from build123d import *

# Parameters (mm, degrees)
CUT_EXTRUDE3_START = 21
CUT_EXTRUDE3_DEPTH = 6.2


with BuildPart() as part:
    # Sketch1 → Revolve1 (revolve)
    with BuildSketch(Plane.XY, mode=Mode.PRIVATE) as revolve1_sk:
        with BuildLine():
            Line((24.3, 17.078694854), (5.260372827, 17.078694854))
            Line((5.260372827, 17.078694854), (5.260372827, 16.028694854))
            Line((5.260372827, 16.028694854), (3.960372827, 16.028694854))
            Line((3.960372827, 16.028694854), (3.960372827, 17.078694854))
            Line((3.960372827, 17.078694854), (-0.7, 17.078694854))
            Line((-0.7, 17.078694854), (-0.7, 2.078694854))
            Line((-0.7, 2.078694854), (295.3, 2.078694854))
            Line((295.3, 2.078694854), (295.3, 17.078694854))
            Line((295.3, 17.078694854), (290.659722162, 17.078694854))
            Line((290.659722162, 17.078694854), (290.659722162, 16.028694854))
            Line((290.659722162, 16.028694854), (289.359722162, 16.028694854))
            Line((289.359722162, 16.028694854), (289.359722162, 17.078694854))
            Line((289.359722162, 17.078694854), (270.3, 17.078694854))
            Line((270.3, 17.078694854), (270.3, 19.578694854))
            Line((270.3, 19.578694854), (229.3, 19.578694854))
            Line((229.3, 19.578694854), (229.3, 18.528694854))
            Line((229.3, 18.528694854), (228, 18.528694854))
            Line((228, 18.528694854), (228, 19.578694854))
            Line((228, 19.578694854), (178, 19.578694854))
            Line((178, 19.578694854), (178, 22.078694854))
            Line((178, 22.078694854), (76.4, 22.078694854))
            Line((76.4, 22.078694854), (76.4, 19.578694854))
            Line((76.4, 19.578694854), (36.4, 19.578694854))
            Line((36.4, 19.578694854), (36.4, 18.728694854))
            ThreePointArc((36.4, 18.728694854), (36.341421356, 18.587273498), (36.2, 18.528694854))
            Line((36.2, 18.528694854), (35.2, 18.528694854))
            ThreePointArc((35.2, 18.528694854), (35.058578644, 18.587273498), (35, 18.728694854))
            Line((35, 18.728694854), (35, 19.578694854))
            Line((35, 19.578694854), (24.3, 19.578694854))
            Line((24.3, 19.578694854), (24.3, 17.078694854))
        make_face()
    revolve(revolve1_sk.sketch.rotate(Axis((-34.240282719, 2.078694854, 0), (1, 0, 0)), 180), axis=Axis((-34.240282719, 2.078694854, 0), (1, 0, 0)))

    # Sketch4 → Cut-Extrude3 (cut)
    with BuildSketch(Plane(origin=(0, 0, 0), x_dir=(1, 0, 0), z_dir=(0, 1, 0)).offset(CUT_EXTRUDE3_START)):
        with BuildLine():
            Line((45.4, 5), (67.4, 5))
            ThreePointArc((67.4, 5), (72.4, 0), (67.4, -5))
            Line((67.4, -5), (45.4, -5))
            ThreePointArc((45.4, -5), (40.4, 0), (45.4, 5))
        make_face()
        with BuildLine():
            Line((192, 5), (214, 5))
            ThreePointArc((214, 5), (219, 0), (214, -5))
            Line((214, -5), (192, -5))
            ThreePointArc((192, -5), (187, 0), (192, 5))
        make_face()
    extrude(amount=-CUT_EXTRUDE3_DEPTH, mode=Mode.SUBTRACT)


solid = part.part
Read the model definition and answer for the solid it produces. Units are mm, in the model's axes. A direction names the side the tool comes from. Round coordinates to 2 decimals unless told otherwise and drop trailing zeros. Order: outer loops, then holes, each group sorted by start corner. A loop starts at its lowest first (then second) coordinate and runs counter-clockwise, first axis right, second up.
1) Flat-ended cylindrical pins translate along their axes: pin 1 (3 mm diameter, centred on x = 202.5, y = 16.5, fed in from -Z); pin 2 (4.5 mm diameter, centred on x = 51.5, y = 16, fed in from +Z); pin 3 (5 mm diameter, centred on x = 49.5, z = -0.5, fed in from +Y). Find the tip coordinate at first contact, or state that the pin passes through.
2) The mould has two halves that part along Z. Classify faces 6 (the face through (292.947, -12.229, -4.506)), 7 (the face through (57, 14.8, 0)), 8 (the face through (5.26, -8, 10)): released by +Z, released by -Z, zero draft, split by the parting line, or undercut.
3) Straight lines are drawn through the part: L1, parallel to X at y = 3, z = -17; L2, parallel to X at y = -7, z = -11.5; L3, parallel to X at y = -7, z = -13. For each, find the intervals that lie inside material, in ascending order.
4) For faces 1 (the face through (219, 17, 0)), 2 (the face through (290.66, -8, 10)), 3 (the face through (270.3, 15, -8)), 4 (the face through (126, -17, -6)), 5 (the face through (24.3, -11, -8)), determine the directions among +Z, -Z, +X, -X, +Y, -Y from which every point of the face is accessible in a straight line to the end or side of a thin tool.
5) The part is cut by section A-A on x = 162.5. Write down the section's boundary in (y, z), plus the area to 3 significant figures.
6) The part is cut by section B-B on x = 260. Write down the section's boundary in (y, z), plus the area to 3 significant figures.
Resolved:
1. pin 1: stops at z = -11.8
1. pin 2: stops at z = 13.04
1. pin 3: stops at y = 14.8
2. face 6: split by the parting line
2. face 7: undercut
2. face 8: zero draft
3. L1: x = 24.3 to 35, 36.4 to 228, 229.3 to 270.3
3. L2: x = -0.7 to 3.96, 5.26 to 289.36, 290.66 to 295.3
3. L3: x = 24.3 to 270.3
4. face 1: +Y
4. face 2: none
4. face 3: +X
4. face 4: +X, -X
4. face 5: -X
5. outline: circle Ø40 at (2.08, 0)
5. area: 1,260 mm2
6. outline: circle Ø35 at (2.08, 0)
6. area: 962 mm2
